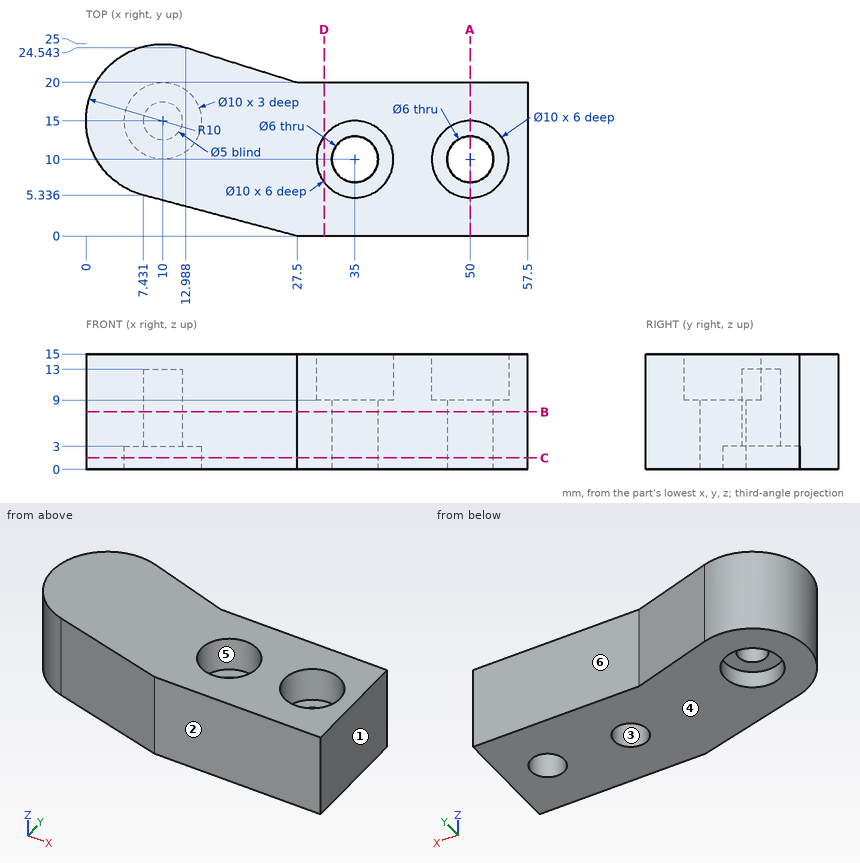
Answer from the drawing. Dimensions are ordinates in mm from the lowest x, y and z of the part. A direction names the side the tool comes from. Coordinates: 2 decimals unless noted, no trailing zeros. Loops run counter-clockwise (first coordinate to the right, second up) from the corner with the lowest first, then second, coordinate; pieces in that order, holes last. Notation, with made-up numbers: (45, -36) - (67, -36) arc R11 ccw to (67, -32) - close; hole circle Ø7 at (42.25, 37). An arc over 180 degrees is marked (long way). Answer in a Markdown table with one row per item.
1. Find section C-C, the plane z = 1.5. Write down the section's boundary in (x, y) (1 decimal), then the cut area to 3 significant figures.
Conclusion:
| item | result |
|---|---|
| outline | (7.4, 5.3) - (27.5, 0) - (57.5, 0) - (57.5, 20) - (27.5, 20) - (13, 24.5) arc R10 ccw (long way) to start; hole circle Ø10 at (10, 15); hole circle Ø6 at (35, 10); hole circle Ø6 at (50, 10) |
| area | 979 mm² |
2. Find section D-D, the plane x = 31. Write down the section's boundary in (y, z).
Conclusion:
| item | result |
|---|---|
| outline | (0, 0) - (20, 0) - (20, 15) - (13, 15) - (13, 9) - (7, 9) - (7, 15) - (0, 15) - close |
3. Find section B-B, the plane z = 7.5. Write down the section's boundary in (x, y) (1 decimal), then the cut area to 3 significant figures.
Conclusion:
| item | result |
|---|---|
| outline | (7.4, 5.3) - (27.5, 0) - (57.5, 0) - (57.5, 20) - (27.5, 20) - (13, 24.5) arc R10 ccw (long way) to start; hole circle Ø5 at (10, 15); hole circle Ø6 at (35, 10); hole circle Ø6 at (50, 10) |
| area | 1,040 mm² |
4. Which of the six approach directions +Z, -Z, +X, -X, +Y, -Y give full straight-line access (tool end or side, diameter ignored) to the marked faces 4, 5 and 6?
Conclusion:
| item | result |
|---|---|
| face 4 | -Z, +X, -X, +Y, -Y |
| face 5 | +Z |
| face 6 | +Z, -Z, +X, +Y |
5. Straight lines are drawn through the part: line 1 (Y direction, x = 50, z = 13.25); line 2 (X direction, y = 10.75, z = 8) (1 decimal); line 3 (Y direction, x = 35, z = 6.5). For each, find the intervals that lie inside material, in ascending order.
Conclusion:
| item | result |
|---|---|
| line 1 | y = 0 to 5, 15 to 20 |
| line 2 | x = 0.9 to 32.1, 37.9 to 47.1, 52.9 to 57.5 |
| line 3 | y = 0 to 7, 13 to 20 |
6. Determine the mould class of the marked faces 1, 2 and 3 for opening direction X: +X half, -X half, draft (parallel to the pull), parting line (faces both ways), or undercut.
Conclusion:
| item | result |
|---|---|
| face 1 | +X half |
| face 2 | draft |
| face 3 | undercut |
7. Find section A-A, the plane x = 50. Write down the section's boundary in (y, z).
Conclusion:
| item | result |
|---|---|
| outline | (0, 0) - (7, 0) - (7, 9) - (5, 9) - (5, 15) - (0, 15) - close; (13, 0) - (20, 0) - (20, 15) - (15, 15) - (15, 9) - (13, 9) - close |
8. Given pin 1 (1 mm diameter, centred on x = 25, z = 10, fed in from +Y); pin 2 (3 mm diameter, centred on x = 35.5, y = 8, fed in from +Z); pin 3 (4 mm diameter, centred on x = 9.5, y = 15.5, fed in from -Z); pin 4 (3.5 mm diameter, centred on x = 35, y = 10, fed in from -Z), each flat-ended and moving along its own axis, determine where each tip first touches the part or whether it passes through.
Conclusion:
| item | result |
|---|---|
| pin 1 | stops at y = 20.94 |
| pin 2 | stops at z = 9 |
| pin 3 | stops at z = 3 |
| pin 4 | passes through |
